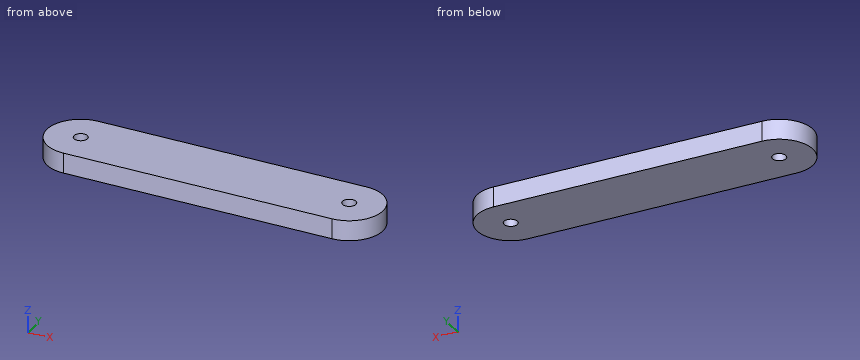
Autodesk Inventor part; units mm, degrees
ref_plane "YZ Plane" through (0, 0, 0) normal (1, 0, 0) x (0, 1, 0)
ref_plane "XZ Plane" through (0, 0, 0) normal (0, 1, 0) x (-1, 0, 0)
ref_plane "XY Plane" through (0, 0, 0) normal (0, 0, 1) x (1, 0, 0)
sketch "スケッチ1" plane through (0, 0, 0) normal (0, 0, 1) x (1, 0, 0)
  line L0 (-100, 25) -> (100, 25)
  line L1 (100, 25) -> (100, -25)
  line L2 (100, -25) -> (-100, -25)
  line L3 (-100, -25) -> (-100, 25)
  arc A0 (-100, 25) -> (-100, -25) centre (-100, 0) ccw
  arc A1 (100, -25) -> (100, 25) centre (100, 0) ccw
  point P0 (0, 0)
  dimension "d0" = 200
  dimension "d1" = 50
  dimension "d2" = 25
  dimension "d3" = 100
extrude "押し出し1" add sketch "スケッチ1" along normal mid plane 15
sketch "スケッチ2" plane through (0, 0, 7.5) normal (0, 0, 1) x (1, 0, 0)
  line L0 (100, 25) -> (-100, 25)
  line L1 (-100, -25) -> (100, -25)
  arc A0 (-100, 25) -> (-100, -25) centre (-100, 0) ccw
  arc A1 (100, -25) -> (100, 25) centre (100, 0) ccw
  circle A2 centre (-100, 0) radius 5
  circle A3 centre (100, 0) radius 5
  point P0 (0, 0)
  dimension "d6" = 10
  dimension "d7" = 10
extrude "押し出し2" cut sketch "スケッチ2" against normal through all contours A2 | A3
properties part number "Arm1" material "アルミニウム 6061"
The model under review builds one solid part; all positions refer to its coordinate system, in mm. Give positions to 0.01 mm unless a question says otherwise; leave off trailing zeros. Write each loop counter-clockwise with the first axis right and the second up, starting at its lowest first coordinate (ties: lowest second). Pieces come first, ordered by that corner, then holes.
(1) Consider section C-C, the plane y = 10.5. Give the boundary of the cut face in (x, z), and give its area (3 significant figures).
(2) Consider section B-B, the plane z = 1. Give the boundary of the cut face in (x, y), and give its area (3 significant figures).
(3) Consider section A-A, the plane y = 0. Give the boundary of the cut face in (x, z).
(4) To check wall thickness, follow L1, parallel to Y at x = 100, z = -3.75; L2, parallel to X at y = 17.5, z = 0.75; L3, parallel to X at y = -22, z = 1.5. State the ranges of each line that lie inside material, in increasing order.
(5) For P1, Ø9, axis at x = -100, y = 0, coming from the +Z side; P2, Ø3, axis at y = 13.5, z = -3, coming from the -X side; P3, Ø2, axis at y = -17.5, z = -5, coming from the +X side, all flat-tipped, find the tip position at first contact; note any pin that passes through.
Returned:
1. outline: (-122.69, -7.5) - (122.69, -7.5) - (122.69, 7.5) - (-122.69, 7.5) - close
1. area: 3,680 mm2
2. outline: (-100, -25) - (100, -25) arc R25 ccw to (100, 25) - (-100, 25) arc R25 ccw to start; hole circle Ø10 at (-100, 0); hole circle Ø10 at (100, 0)
2. area: 11,800 mm2
3. outline: (-125, -7.5) - (-105, -7.5) - (-105, 7.5) - (-125, 7.5) - close; (-95, -7.5) - (95, -7.5) - (95, 7.5) - (-95, 7.5) - close; (105, -7.5) - (125, -7.5) - (125, 7.5) - (105, 7.5) - close
4. L1: y = -25 to -5, 5 to 25
4. L2: x = -117.85 to 117.85
4. L3: x = -111.87 to 111.87
5. P1: passes through
5. P2: stops at x = -121.93
5. P3: stops at x = 118.78
